Model file for the job. Use its own axes, mm. A direction names the side the tool comes from. Coordinates: 2 decimals unless noted, no trailing zeros. Write each loop counter-clockwise with the first axis right and the second up, starting at its lowest first coordinate (ties: lowest second). Pieces come first, ordered by that corner, then holes. Notation, with made-up numbers: M -0.5,24.25 L 47.5,24.25 A22 ccw 47.5,31.25 Z; hole C 66,75.5 d6. An arc over 180 degrees is marked long. Use CSV: the item, a comma, the result in double quotes. Start each with the question number.
from build123d import *

# Parameters (mm, degrees)
F1_DEPTH = 3
F2_R     = 4.25
F3_DEPTH = 7
F4_T     = 1.75
F6_R     = 1.2


# Not quite as in the source:
# - a fillet or chamfer that OpenCascade refuses, or shapes differently, is made with other operations: its cross-section is extruded or revolved along the edge and cut away or added


with BuildPart() as f1:
    # F0 (on Right) → F1 (new body)
    with BuildSketch(Plane.YZ):
        Polygon((-3.25, -1.5), (3.25, -1.5), (3.25, 1.5), (0, 1.5), (-3.25, 1.5), align=None)
    extrude(amount=F1_DEPTH)

    # F2 (on face) → F3 (join)
    with BuildSketch(Plane.XY.offset(1.5)):
        with Locations((1.5, 0)):
            Circle(F2_R)
    extrude(amount=F3_DEPTH)

    # F4
    f4_openings = [f1.faces().sort_by_distance(p)[0] for p in [
        (1.5, 0, -1.5),
        (1.5, 0, 8.5),
    ]]
    offset(amount=F4_T, openings=f4_openings, kind=Kind.INTERSECTION)

    # F5: fillet of radius 1.5 on 1 edges, made by hand


with BuildPart() as f5_tool2:
    # F5_s3 → F5_t4 (revolve)
    with BuildSketch(Plane.XZ):
        with BuildLine():
            ThreePointArc((7.5, 1.25), (7.0606601718, 0.1893398282), (6, -0.25))
            Line((6, -0.25), (7.5, -0.25))
            Line((7.5, -0.25), (7.5, 1.25))
        make_face()
    revolve(axis=Axis((1.5, 0, -0.25), (0, 0, -1)))

    split(bisect_by=Plane.YZ.offset(4.75), keep=Keep.TOP)


with BuildPart() as f1_1:
    add(f1.part)

    # F5_t1: cut F5_tool2
    add(f5_tool2.part, mode=Mode.SUBTRACT)


with BuildPart() as f5_tool7:
    # F5_s8 → F5_t9 (revolve)
    with BuildSketch(Plane.XZ):
        with BuildLine():
            ThreePointArc((7.5, 1.25), (7.0606601718, 0.1893398282), (6, -0.25))
            Line((6, -0.25), (7.5, -0.25))
            Line((7.5, -0.25), (7.5, 1.25))
        make_face()
    revolve(axis=Axis((1.5, 0, -0.25), (0, 0, -1)))

    split(bisect_by=Plane.YZ.offset(-1.75), keep=Keep.BOTTOM)


with BuildPart() as f1_2:
    add(f1_1.part)

    # F5_t6: cut F5_tool7
    add(f5_tool7.part, mode=Mode.SUBTRACT)


with BuildPart() as f5_tool12:
    # F5_s13 → F5_t14 (revolve)
    with BuildSketch(Plane.XZ):
        with BuildLine():
            ThreePointArc((7.5, 1.25), (7.0606601718, 0.1893398282), (6, -0.25))
            Line((6, -0.25), (7.5, -0.25))
            Line((7.5, -0.25), (7.5, 1.25))
        make_face()
    revolve(axis=Axis((1.5, 0, -0.25), (0, 0, -1)))

    split(bisect_by=Plane.XZ.offset(5), keep=Keep.TOP)


with BuildPart() as f1_3:
    add(f1_2.part)

    # F5_t11: cut F5_tool12
    add(f5_tool12.part, mode=Mode.SUBTRACT)


with BuildPart() as f5_tool17:
    # F5_s18 → F5_t19 (revolve)
    with BuildSketch(Plane.XZ):
        with BuildLine():
            ThreePointArc((7.5, 1.25), (7.0606601718, 0.1893398282), (6, -0.25))
            Line((6, -0.25), (7.5, -0.25))
            Line((7.5, -0.25), (7.5, 1.25))
        make_face()
    revolve(axis=Axis((1.5, 0, -0.25), (0, 0, -1)))

    split(bisect_by=Plane.XZ.offset(-5), keep=Keep.BOTTOM)


with BuildPart() as f1_4:
    add(f1_3.part)

    # F5_t16: cut F5_tool17
    add(f5_tool17.part, mode=Mode.SUBTRACT)

    # F6
    f6_edges = [f1_4.edges().sort_by_distance(p)[0] for p in [
        (1.5, 5, -1.5),
        (4.75, 0, -1.5),
        (1.5, -5, -1.5),
        (-1.75, 0, -1.5),
    ]]
    fillet(f6_edges, radius=F6_R)


solid = f1_4.part
1) Band-saw the part on B-B on y = 0. List the corners of the cut face in (x, z).
2) Band-saw the part on C-C on z = 6.5. List the corners of the cut face in (x, y).
3) Tool access for faces 4 (the face through (-1.632, 2.872, 4.951)), 5 (the face through (-2, 0, -0.25)), 6 (the face through (3, 0, 0)): list every direction of +Z, -Z, +X, -X, +Y, -Y with a clear straight run to the whole face (end or side of a thin tool).
4) Two-plate mould, pull along X, no slides. Class faces 1 (the face through (1.454, -4.658, -1.139)), 2 (the face through (4.408, 0.07, -1.139)), 3 (the face through (1, 3.25, 0)): pulls with the +X half, pulls with the -X half, needs draft (parallel to the pull), parting line crosses it, or undercut.
5) Drop flat-ended pins along their axis: P1, Ø5, axis at x = 1.5, y = 0, coming from the +Z side; P2, Ø0.6, axis at x = 5.5, y = -1.5, coming from the -Z side; P3, Ø1.5, axis at x = 2, z = 0, coming from the -Y side; P4, Ø3.5, axis at y = 0.5, z = 0, coming from the -X side. Give the stop position or say it passes through.
6) Band-saw the part on A-A on x = 1.5. List the corners of the cut face in (y, z).
7) Wall check: L1, parallel to Y at x = 1.5, z = 4; L2, parallel to X at y = 3, z = 1; L3, parallel to Y at x = 0.5, z = 6. Give the ranges that are in metal, low to high. Write a range as [from, to].
Findings below:
1,outline,"M -4.5,1.25 A1.5 ccw -3,-0.25 L -1.75,-0.25 L -1.75,-0.3 A1.2 ccw -0.55,-1.5 L 0,-1.5 L 0,1.5 L -2.75,1.5 L -2.75,8.5 L -4.5,8.5 Z; M 3,-1.5 L 3.55,-1.5 A1.2 ccw 4.75,-0.3 L 4.75,-0.25 L 6,-0.25 A1.5 ccw 7.5,1.25 L 7.5,8.5 L 5.75,8.5 L 5.75,1.5 L 3,1.5 Z"
2,outline,"C 1.5,0 d12; hole C 1.5,0 d8.5"
3,face 4,"+Z"
3,face 5,"-Z, -X, +Y, -Y"
3,face 6,"+Z, -Z"
4,face 1,"needs draft"
4,face 2,"pulls with the +X half"
4,face 3,"undercut"
5,P1,"stops at z = 1.5"
5,P2,"stops at z = -0.25"
5,P3,"stops at y = -5.9"
5,P4,"stops at x = -4.5"
6,outline,"M -6,1.25 A1.5 ccw -5,-0.16 L -5,-0.3 A1.2 ccw -3.8,-1.5 L -3.25,-1.5 L -3.25,1.5 L -4.25,1.5 L -4.25,8.5 L -6,8.5 Z; M 3.25,-1.5 L 3.8,-1.5 A1.2 ccw 5,-0.3 L 5,-0.16 A1.5 ccw 6,1.25 L 6,8.5 L 4.25,8.5 L 4.25,1.5 L 3.25,1.5 Z"
7,L1,"y = [-6, -4.25], [4.25, 6]"
7,L2,"x = [-3.67, 0], [3, 6.67]"
7,L3,"y = [-5.92, -4.13], [4.13, 5.92]"
